Verification items for the finished model (mm, model axes). Face numbers are marked on the shaded views. A direction names the side the tool comes from. Round coordinates to 2 decimals unless told otherwise and drop trailing zeros. Write each loop counter-clockwise with the first axis right and the second up, starting at its lowest first coordinate (ties: lowest second). Pieces come first, ordered by that corner, then holes. Notation, with made-up numbers: M 78.5,-5.75 L 135.5,-5.75 A38 ccw 135.5,32.25 Z; hole C 86,50.5 d9. An arc over 180 degrees is marked long. One line per item, written item: value. Start each with the question number.
Item 1: Section check D-D, the plane y = 16. Record the cut outline in (x, z).
Item 2: Gauge pin test, flat end, axial feed: pin 1 (8 mm diameter, centred on y = 5, z = -1.5, fed in from +X). Record the tip position at first contact, or that the pin passes through.
Item 3: Section check A-A, the plane x = -6. Record the cut outline in (y, z).
Item 4: Section check B-B, the plane z = -2. Record the cut outline in (x, y).
Item 5: Section check C-C, the plane x = 9. Record the cut outline in (y, z), then the cut area to 3 significant figures.
Item 6: Thickness scan on probe 1 along Z at (x, y) = (-11.5, 3.5); probe 2 along X at (y, z) = (23.35, -2); probe 3 along Y at (x, z) = (1.5, 0.5). Record the ranges inside material, lowest first. Write a range as from..to.
Item 7: Tool access check on the marked faces 1 and 2. Record the directions out of +Z, -Z, +X, -X, +Y, -Y that give a thin tool (end or side, any length) a straight path to the whole face; none if there is none.
Item 8: Draft check along Z on the marked faces 3, 4 and 5. Enter one of: +Z half, -Z half, draft (parallel to the pull), parting line (faces both ways), or undercut.
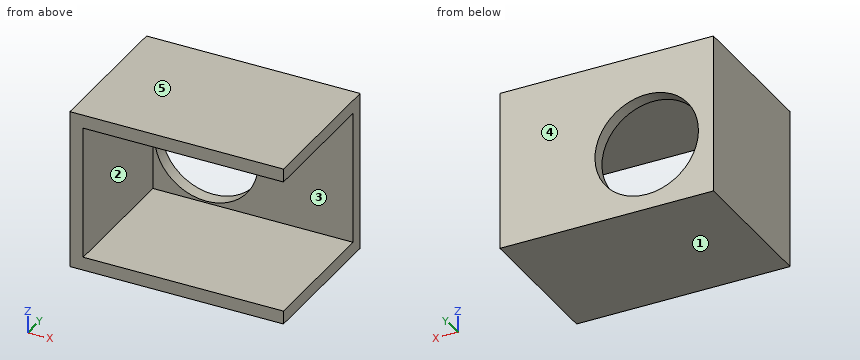
from build123d import *

# Parameters (mm, degrees)
CROQUIS1_W              = 32
CROQUIS1_H              = 24
SALIENTE_EXTRUIR1_DEPTH = 24
VACIADO1_T              = -2
CROQUIS2_R              = 7.75
CORTAR_EXTRUIR1_DEPTH   = 5
CROQUIS3_W              = 32
CROQUIS3_H              = 24
CORTAR_EXTRUIR2_DEPTH   = 2


with BuildPart() as part:
    # Croquis1 → Saliente-Extruir1 (new body)
    with BuildSketch(Plane(origin=(0, 0, 0), x_dir=(1, 0, 0), z_dir=(0, 1, 0))):
        Rectangle(CROQUIS1_W, CROQUIS1_H)
    extrude(amount=SALIENTE_EXTRUIR1_DEPTH)

    # Vaciado1
    vaciado1_openings = [part.faces().sort_by_distance(p)[0] for p in [
        (16, 12, 0),
    ]]
    offset(amount=VACIADO1_T, openings=vaciado1_openings, kind=Kind.INTERSECTION)

    # Croquis2 → Cortar-Extruir1 (cut)
    with BuildSketch(Plane(origin=(0, 22, 0), x_dir=(-1, 0, 0), z_dir=(0, -1, 0))):
        with Locations(Location((6, 2, 0), (0, 0, 90))):
            Circle(CROQUIS2_R)
    extrude(amount=-CORTAR_EXTRUIR1_DEPTH, mode=Mode.SUBTRACT)

    # Croquis3 → Cortar-Extruir2 (cut)
    with BuildSketch(Plane(origin=(0, 0, 0), x_dir=(-1, 0, 0), z_dir=(0, -1, 0))):
        Rectangle(CROQUIS3_W, CROQUIS3_H)
    extrude(amount=-CORTAR_EXTRUIR2_DEPTH, mode=Mode.SUBTRACT)


solid = part.part
Response values:
1. outline: M -16,-12 L 16,-12 L 16,-10 L -14,-10 L -14,10 L 16,10 L 16,12 L -16,12 Z
2. pin 1: stops at x = -14
3. outline: M 2,-12 L 24,-12 L 24,-9.75 L 22,-9.75 L 22,-10 L 2,-10 Z; M 2,10 L 22,10 L 22,5.75 L 24,5.75 L 24,12 L 2,12 Z
4. outline: M -16,2 L -14,2 L -14,22 L -13.75,22 L -13.75,24 L -16,24 Z; M 1.75,22 L 16,22 L 16,24 L 1.75,24 Z
5. outline: M 2,-12 L 24,-12 L 24,12 L 2,12 L 2,10 L 22,10 L 22,-10 L 2,-10 Z
5. area: 128 mm2
6. probe 1: z = -12..-10, 10..12
6. probe 2: x = -16..-13.75, 1.75..16
6. probe 3: y = 22..24
7. face 1: -Z, +X, -X, +Y, -Y
7. face 2: +X, -Y
8. face 3: undercut
8. face 4: draft
8. face 5: +Z half
